from build123d import *

# Parameters (mm, degrees)
SKETCH2_W               = 42
SKETCH2_H               = 1.35
CUT_EXTRUDE1_DEPTH      = 10
CUT_EXTRUDE1_DEPTH_BACK = 10
SKETCH3_R               = 5
CUT_EXTRUDE2_DEPTH      = 79.475065146


with BuildPart() as part:
    # Sketch1 → Revolve1 (revolve)
    with BuildSketch(Plane.XY):
        Polygon((7, 8), (49, 8), (51.5, 8), (52, 7.25069297), (52, 0), (-28, 0), (-28, 8.5), (0, 8.5), (0, 8), align=None)
    revolve(axis=Axis((52, 0, 0), (-1, 0, 0)))

    # Sketch2 → Cut-Extrude1 (cut, two sides)
    with BuildSketch(Plane.XY) as cut_extrude1_sk:
        with Locations((28, 7.325)):
            Rectangle(SKETCH2_W, SKETCH2_H)
    extrude(amount=CUT_EXTRUDE1_DEPTH, mode=Mode.SUBTRACT)
    extrude(cut_extrude1_sk.sketch, amount=-CUT_EXTRUDE1_DEPTH_BACK, mode=Mode.SUBTRACT)

    # Sketch3 → Cut-Extrude2 (cut)
    with BuildSketch(Plane(origin=(52, 0, 0), x_dir=(0, 0, -1), z_dir=(1, 0, 0))):
        with Locations(Location((0, 0, 0), (0, 0, 90))):  # turned: the seam where the file's is
            Circle(SKETCH3_R)
    extrude(amount=-CUT_EXTRUDE2_DEPTH, mode=Mode.SUBTRACT)


solid = part.part
Geometry: final body of the model. Coordinates: model frame, mm. A direction names the side the tool comes from. Give positions to 0.01 mm unless a question says otherwise; leave off trailing zeros. Order: outer loops, then holes, each group sorted by start corner. A loop starts at its lowest first (then second) coordinate and runs counter-clockwise, first axis right, second up. Notation, with made-up numbers: (76.25, 66.5) -> (89.25, 66.5) arc R26 ccw to (89.25, 83.5) -> close; hole circle Ø8 at (46.5, 62). An arc over 180 degrees is marked (long way). Answer as a JSON object with one key per item and string values.
Q1. Section A-A (z = 0). Output: boundary loops of the cut face in (x, y), plus the area to 3 significant figures.
Entries:
{"outline": "(-28, -8.5) -> (0, -8.5) -> (0, -8) -> (51.5, -8) -> (52, -7.25) -> (52, -5) -> (-27.48, -5) -> (-27.48, 5) -> (52, 5) -> (52, 7.25) -> (51.5, 8) -> (49, 8) -> (49, 6.65) -> (7, 6.65) -> (7, 8) -> (0, 8) -> (0, 8.5) -> (-28, 8.5) -> close", "area": "456 mm^2"}
Q2. Access query for faces 4 (the flat face through (-28, 0, 0)), 5 (the flat face through (7, 7, 0)), 6 (the flat face through (-27.475, 0, 0)). Directions: +Z, -Z, +X, -X, +Y, -Y. A direction counts if a zero-diameter tool reaches every point of the face in a straight line with its end or side. Return the directions, or none.
Entries:
{"face 4": "+Z, -Z, -X, +Y, -Y", "face 5": "+Z, -Z, +Y", "face 6": "+X"}
Q3. First-contact query: pin 1 (8 mm diameter, centred on x = 41.5, y = 1, fed in from +Z); pin 2 (3 mm diameter, centred on y = 0.5, z = -0.5, fed in from +X); pin 3 (4.5 mm diameter, centred on x = 28, z = -0.5, fed in from +Y); pin 4 (3 mm diameter, centred on y = -5.5, z = 5.5, fed in from +X). Flat tips, straight axial feed; report the tip coordinate or a pass-through.
Entries:
{"pin 1": "stops at z = 8", "pin 2": "stops at x = -27.48", "pin 3": "stops at y = 6.65", "pin 4": "stops at x = 52"}
Q4. Material intervals for probe 1 along Z at (x, y) = (5.5, 0); probe 2 along Z at (x, y) = (-15.5, 2.25); probe 3 along Y at (x, z) = (14.5, 1), sorted ascending.
Entries:
{"probe 1": "z = -8 to -5, 5 to 8", "probe 2": "z = -8.2 to -4.47, 4.47 to 8.2", "probe 3": "y = -7.94 to -4.9, 4.9 to 6.65"}
Q5. Draft query along Y for faces 1 (the cylindrical face through (12.82, -1.08, -4.88)), 2 (the flat face through (49, 7, 0)), 3 (the flat face through (28, 6.65, 0)). Return one class per face: released by +Y, released by -Y, zero draft, split by the parting line, or undercut.
Entries:
{"face 1": "undercut", "face 2": "zero draft", "face 3": "released by +Y"}
Q6. Section B-B (y = 0). Output: boundary loops of the cut face in (x, z), plus the area to 3 significant figures.
Entries:
{"outline": "(-28, -8.5) -> (0, -8.5) -> (0, -8) -> (51.5, -8) -> (52, -7.25) -> (52, -5) -> (-27.48, -5) -> (-27.48, 5) -> (52, 5) -> (52, 7.25) -> (51.5, 8) -> (0, 8) -> (0, 8.5) -> (-28, 8.5) -> close", "area": "513 mm^2"}
Q7. Section C-C (x = 13.5). Output: boundary loops of the cut face in (y, z), plus the area to 3 significant figures.
Entries:
{"outline": "(6.65, -4.45) -> (6.65, 4.45) arc R8 ccw (long way) to start; hole circle Ø10 at (0, 0)", "area": "114 mm^2"}
